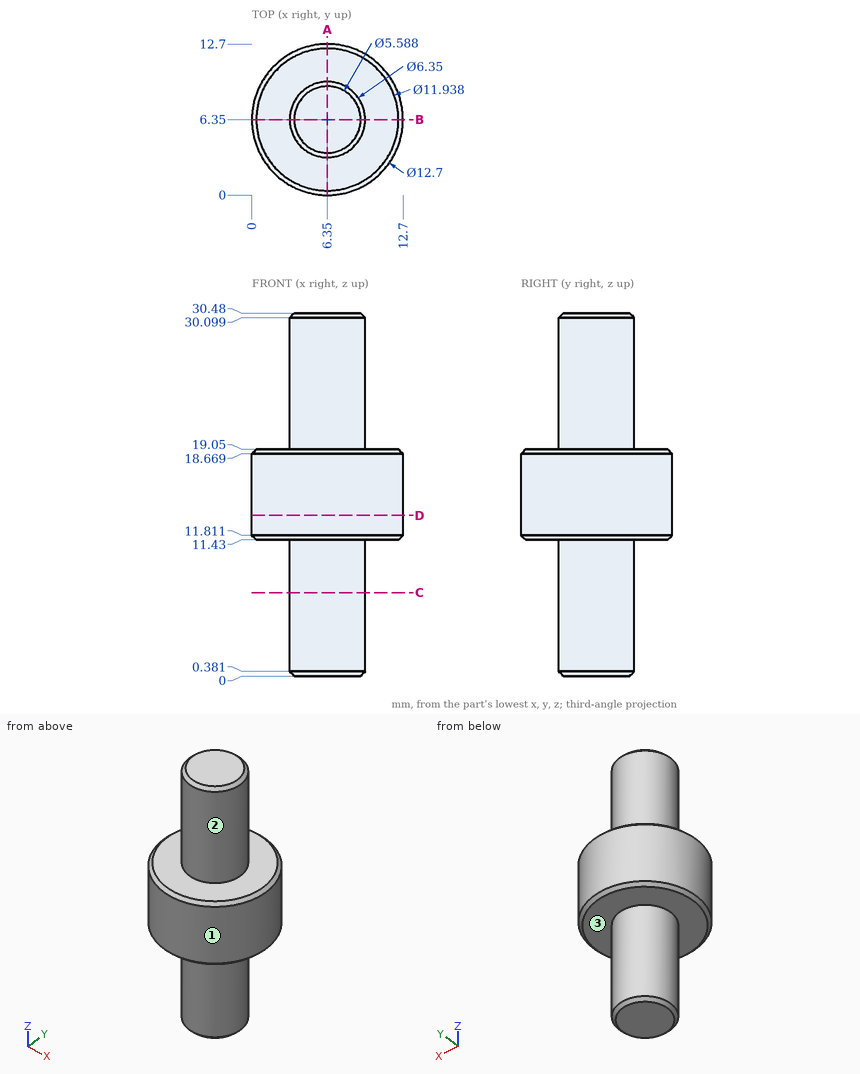
Answer from the drawing. Dimensions are ordinates in mm from the lowest x, y and z of the part. A direction names the side the tool comes from. Give positions to 0.01 mm unless a question says otherwise; leave off trailing zeros. Order: outer loops, then holes, each group sorted by start corner. A loop starts at its lowest first (then second) coordinate and runs counter-clockwise, first axis right, second up.
Item 1: The part is cut by section A-A, the plane x = 6.35. Give the vertices of the cut face in (y, z) (3 decimals).
From the geometry:
outline: (0, 11.811) - (0.381, 11.43) - (3.175, 11.43) - (3.175, 0.381) - (3.556, 0) - (9.144, 0) - (9.525, 0.381) - (9.525, 11.43) - (12.319, 11.43) - (12.7, 11.811) - (12.7, 18.669) - (12.319, 19.05) - (9.525, 19.05) - (9.525, 30.099) - (9.144, 30.48) - (3.556, 30.48) - (3.175, 30.099) - (3.175, 19.05) - (0.381, 19.05) - (0, 18.669) - close
Item 2: The part is cut by section C-C, the plane z = 7. Give the vertices of the cut face in (x, y) (3 decimals).
From the geometry:
outline: circle Ø6.35 at (6.35, 6.35)
Item 3: The part is cut by section D-D, the plane z = 13.5. Give the vertices of the cut face in (x, y).
From the geometry:
outline: circle Ø12.7 at (6.35, 6.35)
Item 4: Which of the six approach directions +Z, -Z, +X, -X, +Y, -Y give full straight-line access (tool end or side, diameter ignored) to the marked faces 1, 2 and 3?
From the geometry:
face 1: +Z, -Z
face 2: +Z
face 3: -Z
Item 5: Find the intervals of material crossed by probe 1 along Z at (x, y) = (5.75, 10.25); probe 2 along X at (y, z) = (6.5, 11); probe 3 along Y at (x, z) = (4, 18.5), in increasing order.
From the geometry:
probe 1: z = 11.43 to 19.05
probe 2: x = 3.18 to 9.52
probe 3: y = 0.45 to 12.25
Item 6: Given pin 1 Ø1 at (y, z) = (8.5, 9.5) entering from +X; pin 2 Ø2 at (x, y) = (8, 10) entering from +Z; pin 3 Ø3 at (x, z) = (2, 19) entering from -Y, each flat-ended and moving along its own axis, determine where each tip first touches the part or whether it passes through.
From the geometry:
pin 1: stops at x = 9.06
pin 2: stops at z = 30.27
pin 3: stops at y = 0.69
